Verification items for this drawing (mm, ordinates from the low corner). A direction names the side the tool comes from. Give positions to 0.01 mm unless a question says otherwise; leave off trailing zeros. Order: outer loops, then holes, each group sorted by start corner. A loop starts at its lowest first (then second) coordinate and runs counter-clockwise, first axis right, second up.
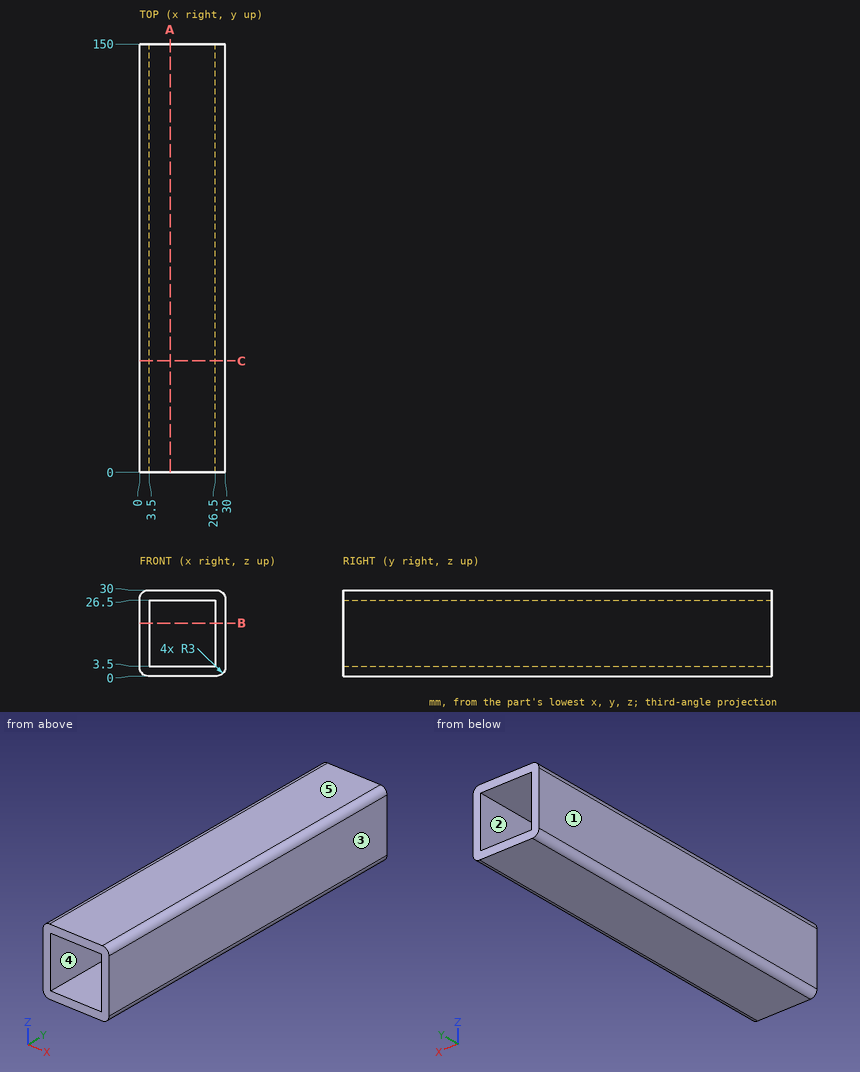
Q1. Cross-section at B-B, the plane z = 18.5. Record the boundary of the cut face in (x, y).
Q2. Thickness scan on L1, parallel to X at y = 10, z = 26; L2, parallel to X at y = 63, z = 1.5. Record the ranges inside material, lowest first.
Q3. Cross-section at C-C, the plane y = 39. Record the boundary of the cut face in (x, z), and give its area (3 significant figures).
Q4. Release check for a two-part mould opening along X. For the marked faces 1, 2 and 3 record: pulls with the +X half, pulls with the -X half, needs draft (parallel to the pull), parting line crosses it, or undercut.
Q5. Access from +Z, -Z, +X, -X, +Y, -Y to the whole of each face (thin tool, end or side, straight path). Record for the marked faces 4 and 5.
Q6. Cross-section at A-A, the plane x = 10.75. Record the boundary of the cut face in (y, z), and give its area (3 significant figures).
Answers follow:
1. outline: (0, 0) - (3.5, 0) - (3.5, 150) - (0, 150) - close; (26.5, 0) - (30, 0) - (30, 150) - (26.5, 150) - close
2. L1: x = 0 to 3.5, 26.5 to 30
2. L2: x = 0.4 to 29.6
3. outline: (0, 3) arc R3 ccw to (3, 0) - (27, 0) arc R3 ccw to (30, 3) - (30, 27) arc R3 ccw to (27, 30) - (3, 30) arc R3 ccw to (0, 27) - close; hole (3.5, 3.5) - (26.5, 3.5) - (26.5, 26.5) - (3.5, 26.5) - close
3. area: 363 mm2
4. face 1: pulls with the -X half
4. face 2: undercut
4. face 3: pulls with the +X half
5. face 4: +Y, -Y
5. face 5: +Z, +X, -X, +Y, -Y
6. outline: (0, 0) - (150, 0) - (150, 3.5) - (0, 3.5) - close; (0, 26.5) - (150, 26.5) - (150, 30) - (0, 30) - close
6. area: 1,050 mm2
